Autodesk Inventor part; units mm, degrees
ref_plane "YZ Plane" through (0, 0, 0) normal (1, 0, 0) x (0, 1, 0)
ref_plane "XZ Plane" through (0, 0, 0) normal (0, 1, 0) x (-1, 0, 0)
ref_plane "XY Plane" through (0, 0, 0) normal (0, 0, 1) x (1, 0, 0)
sketch "스케치1" plane through (0, 0, 0) normal (0, 0, 1) x (1, 0, 0)
  line L0 (-25, 17) -> (25, 17)
  line L1 (25, 17) -> (25, -17)
  line L2 (25, -17) -> (-25, -17)
  line L3 (-25, -17) -> (-25, 17)
  circle A0 centre (0, 0) radius 5.1
  line L4 (0, 0) -> (11, 0)
  line L5 (0, 0) -> (11, 0) construction
  circle A1 centre (11, 0) radius 1.35
  circle A2 centre (7.7782, 7.7782) radius 1.35
  circle A3 centre (0, 11) radius 1.35
  circle A4 centre (-7.7782, 7.7782) radius 1.35
  circle A5 centre (-11, 0) radius 1.35
  circle A6 centre (-7.7782, -7.7782) radius 1.35
  circle A7 centre (0, -11) radius 1.35
  circle A8 centre (7.7782, -7.7782) radius 1.35
  dimension "d0" = 50
  dimension "d1" = 34
  dimension "d2" = 17
  dimension "d3" = 25
  dimension "d4" = 10.2
  dimension "d5" = 11
  dimension "d6" = 0
  dimension "d7" = 2.7
  dimension "d10" = 360
extrude "돌출1" add sketch "스케치1" along normal blind 5
sketch "스케치2" plane through (-25, -17, 0) normal (0, -1, 0) x (1, 0, 0)
  circle A0 centre (4, 2.5) radius 1.25
  circle A1 centre (12, 2.5) radius 1.25
  circle A2 centre (38, 2.5) radius 1.25
  circle A3 centre (46, 2.5) radius 1.25
  line L0 (50, 0) -> (0, 0)
  line L1 (0, 0) -> (0, 5)
  line L2 (50, 0) -> (50, 5)
  point P0 (25, 0)
  dimension "d14" = 2.5
  dimension "d15" = 2.5
  dimension "d16" = 2.5
  dimension "d17" = 2.5
  dimension "d18" = 2.5
  dimension "d19" = 2.5
  dimension "d20" = 2.5
  dimension "d21" = 2.5
  dimension "d22" = 4
  dimension "d23" = 8
  dimension "d24" = 4
  dimension "d25" = 8
extrude "돌출2" cut sketch "스케치2" against normal blind 8
sketch "스케치3" plane through (-25, 17, 0) normal (0, 1, 0) x (1, 0, 0)
  circle A0 centre (38, -2.5) radius 1.25
  circle A1 centre (4, -2.5) radius 1.25
  circle A2 centre (12, -2.5) radius 1.25
  circle A3 centre (46, -2.5) radius 1.25
  line L0 (50, 0) -> (0, 0)
  line L1 (50, 0) -> (50, -5)
  line L2 (0, -5) -> (50, -5)
  line L3 (0, 0) -> (0, -5)
  point P0 (25, 0)
extrude "돌출3" cut sketch "스케치3" against normal blind 8 contours A0 | A1 | A2 | A3
equation "\"d25\" = d23"
properties part number "Box_Top" material "알루미늄 6061"
Can you work these out from the model? Positions are in its coordinate system, mm. A direction names the side the tool comes from. Give positions to 0.01 mm unless a question says otherwise; leave off trailing zeros. Write each loop counter-clockwise with the first axis right and the second up, starting at its lowest first coordinate (ties: lowest second). Pieces come first, ordered by that corner, then holes. Notation, with made-up numbers: (-36.75, 27.25) -> (-20.75, 27.25) arc R31 cw to (-20.75, 59.25) -> close; hole circle Ø6 at (-13, -29). An arc over 180 degrees is marked (long way). One line per item, written item: value.
Q1. Imagine slicing it at A-A on y = 0. Please give me the cut outline in (x, z).
Results found:
outline: (-25, 0) -> (-12.35, 0) -> (-12.35, 5) -> (-25, 5) -> close; (-9.65, 0) -> (-5.1, 0) -> (-5.1, 5) -> (-9.65, 5) -> close; (5.1, 0) -> (9.65, 0) -> (9.65, 5) -> (5.1, 5) -> close; (12.35, 0) -> (25, 0) -> (25, 5) -> (12.35, 5) -> close
Q2. We'd pull the mould along X, two halves only. Please class faces 4 (the face through (0, -17, 2)), 5 (the face through (-25, 0, 2)), 6 (the face through (6.78, 6.87, 2.46)): +X half, -X half, draft (parallel to the pull), parting line (faces both ways), or undercut.
Results found:
face 4: draft
face 5: -X half
face 6: undercut
Q3. Please list where these lines run through material, in increasing order: line 1 (X direction, y = 13, z = 2.5); line 2 (Y direction, x = 0, z = 1.95); line 3 (X direction, y = 7.5, z = 0.6). Write a range as [from, to].
Results found:
line 1: x = [-25, -22.25], [-19.75, -14.25], [-11.75, 11.75], [14.25, 19.75], [22.25, 25]
line 2: y = [-17, -12.35], [-9.65, -5.1], [5.1, 9.65], [12.35, 17]
line 3: x = [-25, -9.1], [-6.46, 6.46], [9.1, 25]
Q4. Which directions (+Z, -Z, +X, -X, +Y, -Y) give clear straight access to the entire face, cutting with the end or side of a thin tool? Please do faces 1 (the face through (22.155, 13.056, 2.979)), 2 (the face through (-19.845, -13.056, 2.021)), 3 (the face through (25, 0, 2)).
Results found:
face 1: +Y
face 2: -Y
face 3: +Z, -Z, +X, +Y, -Y
Q5. Imagine slicing it at B-B on x = 11. Please give me the cut outline in (y, z).
Results found:
outline: (-17, 0) -> (-1.35, 0) -> (-1.35, 5) -> (-17, 5) -> close; (1.35, 0) -> (17, 0) -> (17, 5) -> (1.35, 5) -> close
Q6. Imagine slicing it at D-D on x = 0. Please give me the cut outline in (y, z), and give its area (3 significant figures).
Results found:
outline: (-17, 0) -> (-12.35, 0) -> (-12.35, 5) -> (-17, 5) -> close; (-9.65, 0) -> (-5.1, 0) -> (-5.1, 5) -> (-9.65, 5) -> close; (5.1, 0) -> (9.65, 0) -> (9.65, 5) -> (5.1, 5) -> close; (12.35, 0) -> (17, 0) -> (17, 5) -> (12.35, 5) -> close
area: 92.0 mm^2
Q7. Imagine slicing it at C-C on y = -4. Please give me the cut outline in (x, z), and give its area (3 significant figures).
Results found:
outline: (-25, 0) -> (-3.16, 0) -> (-3.16, 5) -> (-25, 5) -> close; (3.16, 0) -> (25, 0) -> (25, 5) -> (3.16, 5) -> close
area: 218 mm^2
Q8. For P1, Ø1.5, axis at x = -8, y = -8, coming from the -Z side; P2, Ø1.5, axis at x = -13, z = 2.5, coming from the +Y side; P3, Ø2, axis at x = 21, z = 2.5, coming from the -Y side, each with a flat end and sliding along its axis, tell me the tip position at first contact or that it passes through.
Results found:
P1: passes through
P2: stops at y = 9
P3: stops at y = -9
